Work out the finished part from the listing and answer in its coordinate system (mm). Face numbers are marked on the shaded views. A direction names the side the tool comes from. Coordinates: 2 decimals unless noted, no trailing zeros. Write each loop counter-clockwise with the first axis right and the second up, starting at its lowest first coordinate (ties: lowest second). Pieces come first, ordered by that corner, then holes. Notation, with made-up numbers: (56, 10) - (79, 10) arc R17 ccw to (79, 24) - close; hole circle Ø1 at (58.25, 32). An arc over 180 degrees is marked (long way). Use a Markdown table: item, result. Add a question column.
(1) A tool of negligible diameter and unlimited length cuts with its end or side. For the marked faces 1 and 2, from which of +Z, -Z, +X, -X, +Y, -Y can it reach the whole face along a straight path? Write none if from no direction.
(2) The part is cut by section B-B, the plane y = -16. Give the vertices of the cut face in (x, z).
(3) The part is cut by section A-A, the plane x = -17.5. Give the vertices of the cut face in (y, z), then the cut area to 3 significant figures.
(4) For a pull along Z with two mould halves and no side action, classify the marked faces 3, 4, 5 and 6 as released by +Z, released by -Z, zero draft, split by the parting line, or undercut.
(5) Given pin 1 Ø8 at (y, z) = (29.5, 20) entering from -X; pin 2 Ø0.6 at (y, z) = (44, 12.5) entering from -X, each flat-ended and moving along its own axis, determine where each tip first touches the part or whether it passes through.
(6) The part is cut by section C-C, the plane z = -19.5. Give the vertices of the cut face in (x, y).
(7) Find the intervals of material crossed by line 1 (Z direction, x = -11, y = 31.5); line 2 (Y direction, x = -5, z = 4.5); line 3 (X direction, y = -29, z = -21), in increasing order. Write a range as from..to.
Autodesk Inventor part; units mm, degrees
ref_plane "YZ Plane" through (0, 0, 0) normal (1, 0, 0) x (0, 1, 0)
ref_plane "XZ Plane" through (0, 0, 0) normal (0, 1, 0) x (-1, 0, 0)
ref_plane "XY Plane" through (0, 0, 0) normal (0, 0, 1) x (1, 0, 0)
sketch "Esquisse1" plane through (0, 0, 0) normal (1, 0, 0) x (0, 1, 0)
  line L0 (45, 35) -> (-45, 35)
  line L1 (-45, 35) -> (-45, -35)
  line L2 (-45, -35) -> (45, -35)
  line L3 (45, -35) -> (45, 35)
  line L4 (0, 39.01) -> (0, -54.7883) construction
  line L5 (27.6574, 0) -> (-32.6664, 0) construction
  point P0 (0, 0)
  dimension "d0" = 70
  dimension "d1" = 90
extrude "Extrusion1" add sketch "Esquisse1" along normal blind 2
sketch "Esquisse2" plane through (0, 0, 0) normal (-1, 0, 0) x (0, 0, 1)
  line L0 (35, -45) -> (-35, -45)
  line L1 (-35, 45) -> (35, 45)
  line L2 (-35, -45) -> (35, -45)
  line L3 (35, -45) -> (35, 45)
  line L4 (35, 45) -> (-35, 45)
  line L5 (-35, 45) -> (-35, -45)
  line L6 (-33, -43) -> (33, -43)
  line L7 (33, -43) -> (33, 43)
  line L8 (33, 43) -> (-33, 43)
  line L9 (-33, 43) -> (-33, -43)
  point P0 (0, 0)
  dimension "d4" = 2
  dimension "d5" = 2
  dimension "d6" = 2
  dimension "d7" = 2
extrude "Extrusion2" add sketch "Esquisse2" along normal blind 30
fillet "Congé1" radius 2 2 edges at (-14, 45, 35) (-14, -45, 35)
fillet "Congé2" radius 2 2 edges at (-14, 45, -35) (-14, -45, -35)
sketch "Esquisse11" plane through (-30, 45, 33) normal (0, 1, 0) x (1, 0, 0)
  line L0 (0, 66) -> (0, 0)
  line L1 (30, 66) -> (0, 66)
  line L2 (0, 0) -> (3, 0)
  line L3 (3, 0) -> (3, 66)
  line L4 (3, 66) -> (0, 66)
  line L5 (0, 66) -> (0, 0)
  point P0 (30, 33)
  dimension "d79" = 3
extrude "Extrusion11" cut sketch "Esquisse11" against normal blind 10
properties part number "Base"
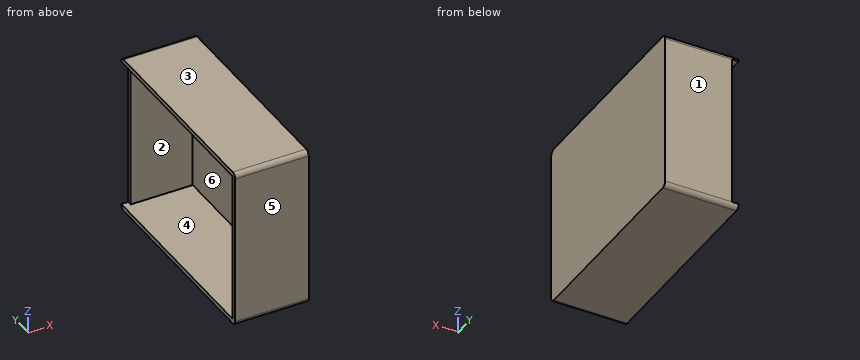
Model answer:
| question | item | result |
|---|---|---|
| 1 | face 1 | +Z, -Z, +X, -X, +Y |
| 1 | face 2 | -X |
| 2 | outline | (-30, -35) - (2, -35) - (2, 35) - (-30, 35) - (-30, 33) - (0, 33) - (0, -33) - (-30, -33) - close |
| 3 | outline | (-45, -33) arc R2 ccw to (-43, -35) - (43, -35) arc R2 ccw to (45, -33) - (45, 33) arc R2 ccw to (43, 35) - (-43, 35) arc R2 ccw to (-45, 33) - close; hole (-43, -33) - (43, -33) - (43, 33) - (-43, 33) - close |
| 3 | area | 621 mm^2 |
| 4 | face 3 | released by +Z |
| 4 | face 4 | undercut |
| 4 | face 5 | zero draft |
| 4 | face 6 | undercut |
| 5 | pin 1 | x = 0 |
| 5 | pin 2 | x = -27 |
| 6 | outline | (-30, -45) - (2, -45) - (2, 45) - (-27, 45) - (-27, 43) - (0, 43) - (0, -43) - (-30, -43) - close |
| 7 | line 1 | -35..-33, 33..35 |
| 7 | line 2 | -45..-43, 43..45 |
| 7 | line 3 | 0..2 |
